Job drawing, mm, ordinate dimensions from the low corner. One solid piece. A direction names the side the tool comes from. Round coordinates to 2 decimals unless told otherwise and drop trailing zeros. Loops run counter-clockwise (first coordinate to the right, second up) from the corner with the lowest first, then second, coordinate; pieces in that order, holes last. Notation, with made-up numbers: (-29, 3.5) - (1, 3.5) arc R11 ccw to (1, 23.5) - close; hole circle Ø2 at (44, -10). An arc over 180 degrees is marked (long way). One line per question, with ' | ' between items. Start each with the question number.
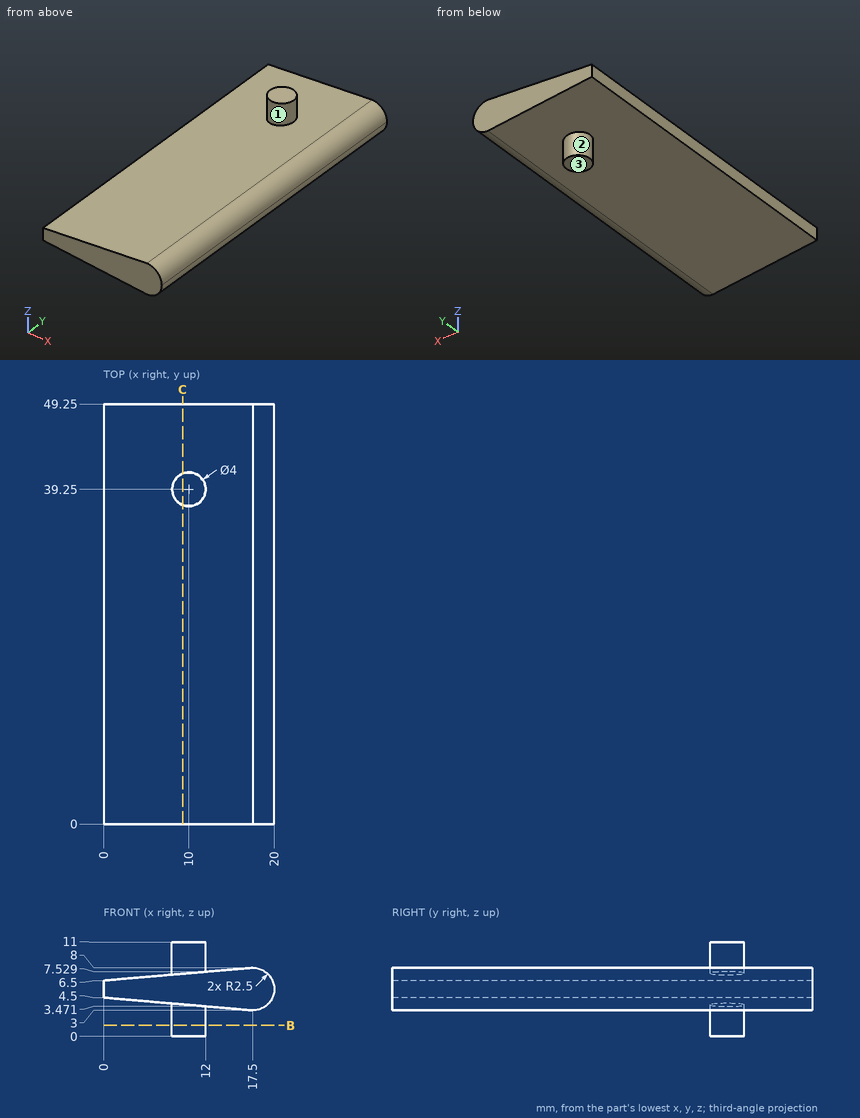
1) Saw through at C-C on x = 9.25. Write the cut outline in (y, z).
2) Saw through at B-B on z = 1.25. Write the cut outline in (x, y).
3) Wall check: line 1 (Z direction, x = 17.5, y = 4); line 2 (Z direction, x = 11, y = 16.5); line 3 (X direction, y = 13, z = 4.75) (1 decimal). Give the ranges that are in metal, low to high. Write a range as [from, to].
4) Tool access for the marked faces 1, 2 and 3: list every direction of +Z, -Z, +X, -X, +Y, -Y with a clear straight run to the whole face (end or side of a thin tool).
5) Drop flat-ended pins along their axis: pin 1 (6 mm diameter, centred on y = 6, z = 4.5, fed in from +X); pin 2 (1.5 mm diameter, centred on x = 4, z = 3, fed in from -Y); pin 3 (2 mm diameter, centred on x = 10, y = 16.5, fed in from -Z); pin 4 (4 mm diameter, centred on y = 31, z = 8.5, fed in from +X). Give the stop position or say it passes through.
Answer key:
1) outline: (0, 3.71) - (37.4, 3.71) - (37.4, 0) - (41.1, 0) - (41.1, 3.71) - (49.25, 3.71) - (49.25, 7.29) - (41.1, 7.29) - (41.1, 11) - (37.4, 11) - (37.4, 7.29) - (0, 7.29) - close
2) outline: circle Ø4 at (10, 39.25)
3) line 1: [3, 8] | line 2: [3.56, 7.44] | line 3: [0, 19.9]
4) face 1: +Z | face 2: -Z | face 3: -Z, +X, -X, +Y, -Y
5) pin 1: x = 20 | pin 2: through | pin 3: z = 3.56 | pin 4: x = 19.79
